Solid Edge part; units mm, degrees
sketch "Sketch1" plane through (0, 0, 0) normal (0, -1, 0) x (1, 0, 0)
  line L0 (45.1982, 14.9945) -> (45.1982, -3.0055)
  line L1 (45.1982, -3.0055) -> (40.1982, -3.0055)
  line L2 (40.1982, -3.0055) -> (40.1982, 4.9945)
  line L3 (31.7982, 4.9945) -> (31.7982, -3.0055)
  line L4 (31.7982, -3.0055) -> (-11.4018, -3.0055)
  line L5 (-11.4018, 4.9945) -> (-11.4018, -3.0055)
  line L6 (-19.8018, 4.9945) -> (-19.8018, -3.0055)
  line L7 (-19.8018, -3.0055) -> (-24.8018, -3.0055)
  line L8 (-24.8018, -3.0055) -> (-24.8018, 14.9945)
  line L9 (-24.8018, 14.9945) -> (45.1982, 14.9945)
  arc A0 (40.1982, 4.9945) -> (31.7982, 4.9945) centre (35.9982, 4.9945) ccw
  arc A1 (-11.4018, 4.9945) -> (-19.8018, 4.9945) centre (-15.6018, 4.9945) ccw
  dimension "D1" = 24.8018
  dimension "D2" = 45.1982
  dimension "D3" = 19.8018
  dimension "D4" = 45.1982
extrude "Protrusion1" add sketch "Sketch1" against normal blind 8
Work out the finished part from the listing and answer in its coordinate system (mm). A direction names the side the tool comes from. Round coordinates to 2 decimals unless told otherwise and drop trailing zeros. Write each loop counter-clockwise with the first axis right and the second up, starting at its lowest first coordinate (ties: lowest second). Pieces come first, ordered by that corner, then holes.
1) A cutting plane is placed at D-D (z = 8). Give the vertices of the cut face in (x, y), plus the area to 3 significant figures.
2) A cutting plane is placed at B-B (y = 4.5). Give the vertices of the cut face in (x, z).
3) A cutting plane is placed at C-C (x = 36). Give the vertices of the cut face in (y, z), plus the area to 3 significant figures.
4) A tool of negligible diameter and unlimited length cuts with its end or side. For faces 4 (the flat face through (-11.402, 4, 1)), 5 (the flat face through (-24.802, 4, 6)), from which of +Z, -Z, +X, -X, +Y, -Y can it reach the whole face along a straight path? Write none if from no direction.
5) The mould has two halves that part along X. Classify faces 1 (the cylindrical face through (36.091, 3.944, 9.193)), 2 (the flat face through (45.198, 4, 6)), 3 (the flat face through (11, 8, 6)): pulls with the +X half, pulls with the -X half, needs draft (parallel to the pull), parting line crosses it, or undercut.
6) Straight lines are drawn through the part: line 1 (X direction, y = 2.75, z = 2); line 2 (X direction, y = 1.75, z = 7); line 3 (Z direction, x = 36, y = 0.5). For each, find the intervals that lie inside material, in ascending order.
7) A cutting plane is placed at A-A (z = 1.5). Give the vertices of the cut face in (x, y).
Completed:
1. outline: (-24.8, 0) - (-18.54, 0) - (-18.54, 8) - (-24.8, 8) - close; (-12.67, 0) - (33.06, 0) - (33.06, 8) - (-12.67, 8) - close; (38.93, 0) - (45.2, 0) - (45.2, 8) - (38.93, 8) - close
1. area: 466 mm2
2. outline: (-24.8, -3.01) - (-19.8, -3.01) - (-19.8, 4.99) arc R4.2 cw to (-11.4, 4.99) - (-11.4, -3.01) - (31.8, -3.01) - (31.8, 4.99) arc R4.2 cw to (40.2, 4.99) - (40.2, -3.01) - (45.2, -3.01) - (45.2, 14.99) - (-24.8, 14.99) - close
3. outline: (0, 9.19) - (8, 9.19) - (8, 14.99) - (0, 14.99) - close
3. area: 46.4 mm2
4. face 4: -Z, +Y, -Y
4. face 5: +Z, -Z, -X, +Y, -Y
5. face 1: undercut
5. face 2: pulls with the +X half
5. face 3: needs draft
6. line 1: x = -24.8 to -19.8, -11.4 to 31.8, 40.2 to 45.2
6. line 2: x = -24.8 to -19.29, -11.91 to 32.31, 39.69 to 45.2
6. line 3: z = 9.19 to 14.99
7. outline: (-24.8, 0) - (-19.8, 0) - (-19.8, 8) - (-24.8, 8) - close; (-11.4, 0) - (31.8, 0) - (31.8, 8) - (-11.4, 8) - close; (40.2, 0) - (45.2, 0) - (45.2, 8) - (40.2, 8) - close
